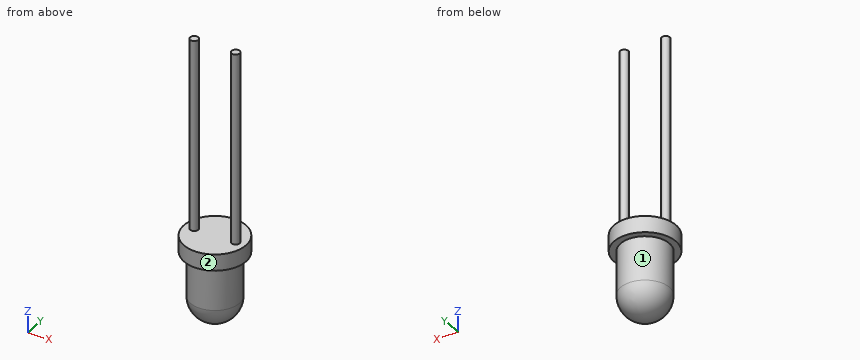
from build123d import *

# Parameters (mm, degrees)
SKETCH_1_R      = 1.5
EXTRUDE_1_DEPTH = 3.7
SKETCH_2_R      = 1.9
EXTRUDE_2_DEPTH = 1
SKETCH_3_R      = 0.25
EXTRUDE_3_DEPTH = 12.7


with BuildPart() as part:
    # 草图1 → 拉伸1 (new body)
    with BuildSketch(Plane.XY):
        Circle(SKETCH_1_R)
    extrude(amount=EXTRUDE_1_DEPTH)

    # 草图2 → 拉伸2 (add)
    with BuildSketch(Plane.XY.offset(3.7)):
        Circle(SKETCH_2_R)
    extrude(amount=-EXTRUDE_2_DEPTH)

    # 草图3 → 拉伸3 (add)
    with BuildSketch(Plane(origin=(0, 0, 2.7), x_dir=(-1, 0, 0), z_dir=(0, 0, -1))):
        with Locations((-1.27, 0)):
            Circle(SKETCH_3_R)
        with Locations(Location((1.27, 0, 0), (0, 0, 180))):
            Circle(SKETCH_3_R)
    extrude(amount=-EXTRUDE_3_DEPTH)

    # 草图5 → 旋转2 (revolve)
    with BuildSketch(Plane(origin=(0, 0, 0), x_dir=(0, 0, -1), z_dir=(1, 0, 0))):
        with BuildLine():
            Line((0, 1.5), (0, 0))
            Line((0, 0), (1.5, 0))
            ThreePointArc((1.5, 0), (1.060660172, 1.060660172), (0, 1.5))
        make_face()
    revolve(axis=Axis((0, 0, -1.5), (0, 0, 1)))


solid = part.part
The listing builds one solid part. Answer for the finished solid, in the listing's coordinates (mm). Face numbers are marked on the shaded views. A direction names the side the tool comes from. Coordinates: 2 decimals unless noted, no trailing zeros. Write each loop counter-clockwise with the first axis right and the second up, starting at its lowest first coordinate (ties: lowest second). Pieces come first, ordered by that corner, then holes. Notation, with made-up numbers: (56.5, -7.75) - (63.5, -7.75) arc R14 ccw to (63.5, -0.75) - close; hole circle Ø10 at (55, -31.5). An arc over 180 degrees is marked (long way). Answer as CSV lines item,"result".
1. Find section A-A (x = 0). Give the vertices of the cut face in (y, z), plus the area to 3 significant figures.
Computed values:
outline,"(-1.9, 2.7) - (-1.5, 2.7) - (-1.5, 0) arc R1.5 ccw to (1.5, 0) - (1.5, 2.7) - (1.9, 2.7) - (1.9, 3.7) - (-1.9, 3.7) - close"
area,"15.4 mm²"
2. Find section C-C (z = 5.5). Give the vertices of the cut face in (x, y).
Computed values:
outline,"circle Ø0.5 at (-1.27, 0); circle Ø0.5 at (1.27, 0)"
3. Find section D-D (y = 1.05). Give the vertices of the cut face in (x, z), plus the area to 3 significant figures.
Computed values:
outline,"(-1.58, 2.7) - (-1.07, 2.7) - (-1.07, 0) arc R1.07 ccw to (1.07, 0) - (1.07, 2.7) - (1.58, 2.7) - (1.58, 3.7) - (-1.58, 3.7) - close"
area,"10.8 mm²"
4. Find section B-B (y = 0). Give the vertices of the cut face in (x, z).
Computed values:
outline,"(-1.9, 2.7) - (-1.5, 2.7) - (-1.5, 0) arc R1.5 ccw to (1.5, 0) - (1.5, 2.7) - (1.9, 2.7) - (1.9, 3.7) - (1.52, 3.7) - (1.52, 15.4) - (1.02, 15.4) - (1.02, 3.7) - (-1.02, 3.7) - (-1.02, 15.4) - (-1.52, 15.4) - (-1.52, 3.7) - (-1.9, 3.7) - close"
5. Given P1, Ø1.9, axis at x = 0, y = 0, coming from the +Z side, flat-ended and moving along its own axis, determine where the tip first touches the part or whether it passes through.
Computed values:
P1,"stops at z = 3.7"
6. A tool of negligible diameter and unlimited length cuts with its end or side. For the marked faces 1 and 2, from which of +Z, -Z, +X, -X, +Y, -Y can it reach the whole face along a straight path? Write none if from no direction.
Computed values:
face 1,"-Z"
face 2,"+Z, -Z"
7. Straight lines are drawn through the part: line 1 (Z direction, x = -1.4, y = -0.8); line 2 (X direction, y = 0.2, z = 4); line 3 (Z direction, x = -0.05, y = 0.85). For each, find the intervals that lie inside material, in ascending order. Write a range as [from, to].
Computed values:
line 1,"z = [2.7, 3.7]"
line 2,"x = [-1.42, -1.12], [1.12, 1.42]"
line 3,"z = [-1.23, 3.7]"
